Part model, mm, in its own coordinate system. A direction names the side the tool comes from. Give positions to 0.01 mm unless a question says otherwise; leave off trailing zeros. Write each loop counter-clockwise with the first axis right and the second up, starting at its lowest first coordinate (ties: lowest second). Pieces come first, ordered by that corner, then holes. Notation, with made-up numbers: M -8.5,80.25 L 42.5,80.25 A19 cw 42.5,112.25 Z; hole C -27,58 d2. An arc over 180 degrees is marked long. Answer as CSV lines item,"result". Start each with the question number.
1) Pin check, flat tips, straight feed: pin 1 Ø1.5 at (x, z) = (4, 7.5) entering from +Y; pin 2 Ø3 at (x, y) = (-3.5, 4.5) entering from +Z; pin 3 Ø1 at (y, z) = (-0.5, 7) entering from +X; pin 4 Ø1.5 at (x, z) = (7, 7) entering from +Y. Stop position of each tip, or through.
2) Slice it at C-C, the plane x = 10.75. Give the cut face in (y, z), plus the area to 3 significant figures.
3) Slice it at A-A, the plane y = 0. Give the cut face in (x, z).
4) Tool access for faces 4 (the flat face through (-12.56, 0, 1)), 5 (the cylindrical face through (4.92, -4.88, 5.61)): list every direction of +Z, -Z, +X, -X, +Y, -Y with a clear straight run to the whole face (end or side of a thin tool).
5) Wall check: line 1 along X through (y, z) = (-0.25, 5.5); line 2 along Z through (x, y) = (8.25, 5.25); line 3 along X through (y, z) = (1, 4). Give the ranges that are in metal, low to high. Write a range as from..to.
6) Mould opens along X. For faces 1 (the cylindrical face through (-4.92, 4.88, 5.61)), 2 (the flat face through (6, 0, 8.298)), 3 (the flat face through (12.56, 0, 1)) say: pulls with the +X half, pulls with the -X half, needs draft (parallel to the pull), parting line crosses it, or undercut.
7) Slice it at D-D, the plane x = -3. Give the cut face in (y, z) (3 decimals), plus the area to 3 significant figures.
8) Slice it at B-B, the plane z = 7.25. Give the cut face in (x, y).
```python
from build123d import *

# Parameters (mm, degrees)
SKETCH_3_W      = 25.120236726
SKETCH_3_H      = 12.02564524
EXTRUDE_1_DEPTH = 3
SKETCH_4_R      = 5
EXTRUDE_2_DEPTH = 5.297900912


with BuildPart() as part:
    # 草图3 → 凸台-拉伸1 (new body)
    with BuildSketch(Plane.XY):
        Rectangle(SKETCH_3_W, SKETCH_3_H)
    extrude(amount=EXTRUDE_1_DEPTH)

    # 草图4 → 凸台-拉伸2 (add)
    with BuildSketch(Plane.XY.offset(3)):
        with Locations((6.006662197, 0)):
            Circle(SKETCH_4_R)
        with Locations(Location((-6.006662197, 0, 0), (0, 0, 180))):
            Circle(SKETCH_4_R)
    extrude(amount=EXTRUDE_2_DEPTH)


solid = part.part
```
Found:
1,pin 1,"y = 4.84"
1,pin 2,"z = 8.3"
1,pin 3,"x = 11.01"
1,pin 4,"y = 4.99"
2,outline,"M -6.01,0 L 6.01,0 L 6.01,3 L 1.58,3 L 1.58,8.3 L -1.58,8.3 L -1.58,3 L -6.01,3 Z"
2,area,"52.8 mm²"
3,outline,"M -12.56,0 L 12.56,0 L 12.56,3 L 11.01,3 L 11.01,8.3 L 1.01,8.3 L 1.01,3 L -1.01,3 L -1.01,8.3 L -11.01,8.3 L -11.01,3 L -12.56,3 Z"
4,face 4,"+Z, -Z, -X, +Y, -Y"
4,face 5,"+Z"
5,line 1,"-11..-1.01, 1.01..11"
5,line 2,"0..3"
5,line 3,"-10.91..-1.11, 1.11..10.91"
6,face 1,"undercut"
6,face 2,"needs draft"
6,face 3,"pulls with the +X half"
7,outline,"M -6.013,0 L 6.013,0 L 6.013,3 L 3.995,3 L 3.995,8.298 L -3.995,8.298 L -3.995,3 L -6.013,3 Z"
7,area,"78.4 mm²"
8,outline,"C -6.01,0 d10; C 6.01,0 d10"
